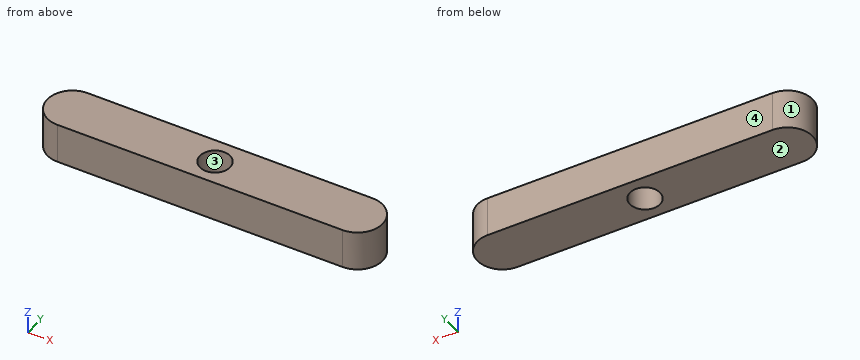
from build123d import *

# Parameters (mm, degrees)
SALIENTE_EXTRUIR1_DEPTH = 2
CROQUIS2_R              = 0.75
CORTAR_EXTRUIR1_DEPTH   = 2


with BuildPart() as part:
    # Croquis1 → Saliente-Extruir1 (new body)
    with BuildSketch(Plane.XY):
        with BuildLine():
            Line((0, -2.5), (0, 0))
            Line((0, 0), (-7, 0))
            ThreePointArc((-7, 0), (-8.25, -1.25), (-7, -2.5))
            Line((-7, -2.5), (0, -2.5))
        make_face()
        with BuildLine():
            Line((7, 0), (0, 0))
            Line((0, 0), (0, -2.5))
            Line((0, -2.5), (7, -2.5))
            ThreePointArc((7, -2.5), (8.25, -1.25), (7, 0))
        make_face()
    extrude(amount=SALIENTE_EXTRUIR1_DEPTH)

    # Croquis2 → Cortar-Extruir1 (cut)
    with BuildSketch(Plane.XY.offset(2)):
        with Locations((0, -1.25)):
            Circle(CROQUIS2_R)
    extrude(amount=-CORTAR_EXTRUIR1_DEPTH, mode=Mode.SUBTRACT)


solid = part.part
Geometry: final body of the model. Coordinates: model frame, mm. Face numbers are marked on the shaded views. Round coordinates to 2 decimals unless told otherwise and drop trailing zeros. Loops run counter-clockwise (first coordinate to the right, second up) from the corner with the lowest first, then second, coordinate; pieces in that order, holes last.
Q1. Section B-B on x = 0. Return loops of the section in (y, z).
Q2. Material intervals for L1, parallel to Y at x = 0, z = 1.1; L2, parallel to X at y = -1.75, z = 1.5; L3, parallel to X at y = -0.95, z = 0.2, sorted ascending.
Q3. Pull-direction query (Y, two-part tool) for the marked faces 1, 2, 3 and 4; classes: released by +Y, released by -Y, zero draft, split by the parting line, or undercut.
Q4. Pin query (flat end, axial travel): P1, Ø1, axis at x = -1, y = -1.5, coming from the -Z side. Return the tip coordinate at first contact, or that it passes through.
Q5. Section C-C on z = 1. Return loops of the section in (x, y).
Q6. Section A-A on y = -1.25. Return loops of the section in (x, z), plus the area to 3 significant figures.
Evaluation:
1. outline: (-2.5, 0) - (-2, 0) - (-2, 2) - (-2.5, 2) - close; (-0.5, 0) - (0, 0) - (0, 2) - (-0.5, 2) - close
2. L1: y = -2.5 to -2, -0.5 to 0
2. L2: x = -8.15 to -0.56, 0.56 to 8.15
2. L3: x = -8.21 to -0.69, 0.69 to 8.21
3. face 1: split by the parting line
3. face 2: zero draft
3. face 3: undercut
3. face 4: released by +Y
4. P1: stops at z = 0
5. outline: (-7, -2.5) - (7, -2.5) arc R1.25 ccw to (7, 0) - (-7, 0) arc R1.25 ccw to start; hole circle Ø1.5 at (0, -1.25)
6. outline: (-8.25, 0) - (-0.75, 0) - (-0.75, 2) - (-8.25, 2) - close; (0.75, 0) - (8.25, 0) - (8.25, 2) - (0.75, 2) - close
6. area: 30.0 mm2
